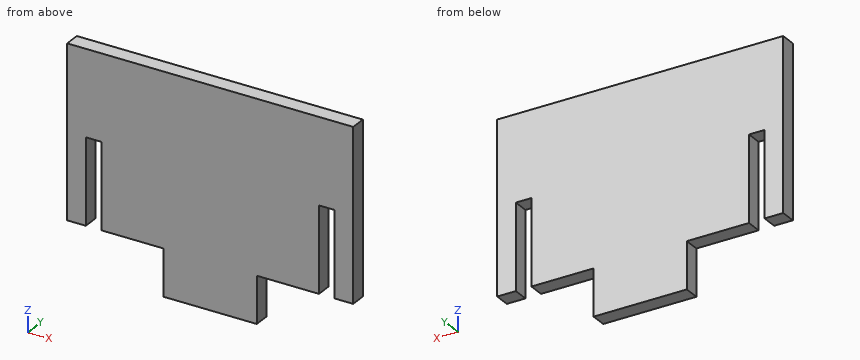
from build123d import *

# Parameters (mm, degrees)
SKETCH1_W           = 92
SKETCH1_H           = 55
BOSS_EXTRUDE1_DEPTH = 2.5
SKETCH2_W           = 5
SKETCH2_H           = 27.5
CUT_EXTRUDE1_DEPTH  = 6
SKETCH3_W           = 29.98
SKETCH3_H           = 15
BOSS_EXTRUDE2_DEPTH = 5


with BuildPart() as part:
    # Sketch1 → Boss-Extrude1 (new body, symmetric)
    with BuildSketch(Plane(origin=(0, 0, 0), x_dir=(1, 0, 0), z_dir=(0, 1, 0))):
        Rectangle(SKETCH1_W, SKETCH1_H)
    extrude(amount=BOSS_EXTRUDE1_DEPTH, both=True)

    # Sketch2 → Cut-Extrude1 (cut, through all)
    with BuildSketch(Plane(origin=(0, 2.5, 0), x_dir=(1, 0, 0), z_dir=(0, 1, 0))):
        with Locations((-37.5, 13.75)):
            Rectangle(SKETCH2_W, SKETCH2_H)
        with Locations((37.5, 13.75)):
            Rectangle(SKETCH2_W, SKETCH2_H)
    extrude(amount=-CUT_EXTRUDE1_DEPTH, mode=Mode.SUBTRACT)

    # Sketch3 → Boss-Extrude2 (add)
    with BuildSketch(Plane(origin=(0, 2.5, 0), x_dir=(1, 0, 0), z_dir=(0, 1, 0))):
        with Locations((0, 35)):
            Rectangle(SKETCH3_W, SKETCH3_H)
    extrude(amount=-BOSS_EXTRUDE2_DEPTH)


solid = part.part
Geometry: final body of the model. Coordinates: model frame, mm. Give positions to 0.01 mm unless a question says otherwise; leave off trailing zeros. Loops run counter-clockwise (first coordinate to the right, second up) from the corner with the lowest first, then second, coordinate; pieces in that order, holes last. Notation, with made-up numbers: M 35,-36 L 65,-36 A23 ccw 65,-8 Z; hole C 47.25,13 d3. An arc over 180 degrees is marked long. Put each result on its own line as item: value. Start each with the question number.
1) Cut plane B-B (y = 1.7). Output: boundary loops of the cut face in (x, z).
2) Contact query for flat-ended pins moving along their axis: pin 1 (2.5 mm diameter, centred on x = 37.5, y = 0.5, fed in from -Z); pin 2 (2.5 mm diameter, centred on x = 26.5, y = 0, fed in from -Z); pin 3 (2.5 mm diameter, centred on y = 1, z = -32, fed in from +X). Output: stop coordinate, or through.
3) Cut plane A-A (z = -19). Output: boundary loops of the cut face in (x, y), then the cut area to 3 significant figures.
4) Cut plane D-D (z = -31). Output: boundary loops of the cut face in (x, y).
5) Cut plane C-C (x = 23.5). Output: boundary loops of the cut face in (y, z), then the cut area to 3 significant figures.
6) Ray query, line 1 along X through (y, z) = (2.15, -9); line 2 along X through (y, z) = (0.85, -34); line 3 along Z through (x, y) = (-15.5, 2.1). Return the intervals inside material, ascending.
Verdict:
1. outline: M -46,-27.5 L -40,-27.5 L -40,0 L -35,0 L -35,-27.5 L -14.99,-27.5 L -14.99,-42.5 L 14.99,-42.5 L 14.99,-27.5 L 35,-27.5 L 35,0 L 40,0 L 40,-27.5 L 46,-27.5 L 46,27.5 L -46,27.5 Z
2. pin 1: z = 0
2. pin 2: z = -27.5
2. pin 3: x = 14.99
3. outline: M -46,-2.5 L -40,-2.5 L -40,2.5 L -46,2.5 Z; M -35,-2.5 L 35,-2.5 L 35,2.5 L -35,2.5 Z; M 40,-2.5 L 46,-2.5 L 46,2.5 L 40,2.5 Z
3. area: 410 mm2
4. outline: M -14.99,-2.5 L 14.99,-2.5 L 14.99,2.5 L -14.99,2.5 Z
5. outline: M -2.5,-27.5 L 2.5,-27.5 L 2.5,27.5 L -2.5,27.5 Z
5. area: 275 mm2
6. line 1: -46 to -40, -35 to 35, 40 to 46
6. line 2: -14.99 to 14.99
6. line 3: -27.5 to 27.5
